Read the model definition and answer for the solid it produces. Units are mm, in the model's axes. Coordinates: 2 decimals unless noted, no trailing zeros. Write each loop counter-clockwise with the first axis right and the second up, starting at its lowest first coordinate (ties: lowest second). Pieces come first, ordered by that corner, then holes. Notation, with made-up numbers: (67, -4) -> (123, -4) arc R11 cw to (123, 11) -> close; hole circle Ø4 at (36, 5). An arc over 180 degrees is marked (long way). One line per item, written item: value. Start each with the question number.
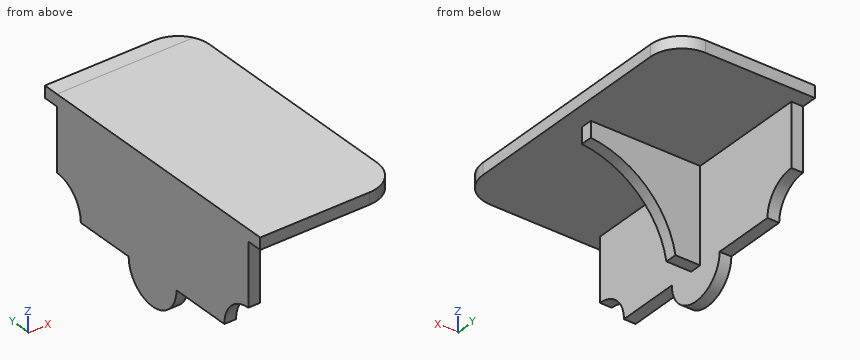
from build123d import *

# Parameters (mm, degrees)
F0_W      = 203.2
F0_H      = 9.525
F0_W_2    = 12.7
F1_DEPTH  = 114.3
F2_DEPTH  = 9.525
F3_W      = 9.525
F3_H      = 76.2
F4_DEPTH  = 88.9
F6_DEPTH  = 119.0635
F8_DEPTH  = 9.526
F10_DEPTH = 9.6059256377


with BuildPart() as f1:
    # F0 (on Right) → F1 (new body)
    with BuildSketch(Plane.YZ):
        with Locations((-2.4829334736, 39.2448874779)):
            Rectangle(F0_W, F0_H)
        Polygon((99.1170665264, 44.0073874779), (99.1170665264, 34.4823874779), (111.8170665264, 34.4823874779), (111.8170665264, 44.0873131156), align=None)
        with Locations((-110.4329334736, 39.2448874779)):
            Rectangle(F0_W_2, F0_H)
    extrude(amount=F1_DEPTH)

    # F0 (on Right) → F2 (join)
    with BuildSketch(Plane.YZ):
        Polygon((99.1170665264, 34.4823874779), (-104.0829334736, 34.4823874779), (-104.0829334736, -41.7176125221), (-27.8829334736, -41.7176125221), (22.9170665264, -41.7176125221), (99.1170665264, -41.7176125221), align=None)
        with BuildLine():
            Line((22.9170665264, -41.7176125221), (-27.8829334736, -41.7176125221))
            ThreePointArc((-27.8829334736, -41.7176125221), (-2.4829334736, -67.1176125221), (22.9170665264, -41.7176125221))
        make_face()
    extrude(amount=F2_DEPTH)

    # F3 (on face) → F4 (join)
    with BuildSketch(Plane.YZ.offset(9.525)):
        with Locations((-2.4829334736, -3.6176125221)):
            Rectangle(F3_W, F3_H)
    extrude(amount=F4_DEPTH)

    # F5 (on face) → F6 (cut, through all)
    with BuildSketch(Plane(origin=(0, 2.2795665264, 0), x_dir=(-1, 0, 0), z_dir=(0, 1, 0))):
        with BuildLine():
            ThreePointArc((-29.6407867546, -41.7176125221), (-53.2038437376, 1.6792308985), (-98.425, 21.5173431966))
            Line((-98.425, 21.5173431966), (-98.425, -41.7176125221))
            Line((-98.425, -41.7176125221), (-29.6407867546, -41.7176125221))
        make_face()
    extrude(amount=-F6_DEPTH, mode=Mode.SUBTRACT)

    # F7 (on face) → F8 (cut, through all)
    with BuildSketch(Plane.YZ.offset(9.525)):
        with BuildLine():
            Line((-104.0829334736, -41.7176125221), (-78.6829334736, -41.7176125221))
            ThreePointArc((-78.6829334736, -41.7176125221), (-86.1224212314, -23.75710028), (-104.0829334736, -16.3176125221))
            Line((-104.0829334736, -16.3176125221), (-104.0829334736, -41.7176125221))
        make_face()
        with BuildLine():
            Line((99.1170665264, -41.7176125221), (99.1170665264, -16.3176125221))
            ThreePointArc((99.1170665264, -16.3176125221), (81.1565542843, -23.75710028), (73.7170665264, -41.7176125221))
            Line((73.7170665264, -41.7176125221), (99.1170665264, -41.7176125221))
        make_face()
    extrude(amount=-F8_DEPTH, mode=Mode.SUBTRACT)

    # F9 (on face) → F10 (cut, through all)
    with BuildSketch(Plane(origin=(0, 0, 34.4823874779), x_dir=(1, 0, 0), z_dir=(0, 0, -1))):
        with BuildLine():
            ThreePointArc((88.9, 116.7829334736), (106.8605122421, 109.3434457157), (114.3, 91.3829334736))
            Line((114.3, 91.3829334736), (114.3, 116.7829334736))
            Line((114.3, 116.7829334736), (89.5812958479, 116.7829334736))
            Line((89.5812958479, 116.7829334736), (88.9, 116.7829334736))
        make_face()
        with BuildLine():
            Line((114.3, -111.8170665264), (114.3, -86.4170665264))
            ThreePointArc((114.3, -86.4170665264), (106.8605122421, -104.3775787686), (88.9, -111.8170665264))
            Line((88.9, -111.8170665264), (95.8859026432, -111.8170665264))
            Line((95.8859026432, -111.8170665264), (114.3, -111.8170665264))
        make_face()
    extrude(amount=-F10_DEPTH, mode=Mode.SUBTRACT)


solid = f1.part
1. A cutting plane is placed at B-B on x = 18.5. Give the vertices of the cut face in (y, z), then the cut area to 3 significant figures.
2. A cutting plane is placed at D-D on z = -8. Give the vertices of the cut face in (x, y) (1 decimal).
3. A cutting plane is placed at C-C on z = 8. Give the vertices of the cut face in (x, y) (3 decimals), then the cut area to 3 significant figures.
4. Given pin 1 (7.5 mm diameter, centred on x = 5.5, z = 18.5, fed in from -Y); pin 2 (1.5 mm diameter, centred on y = -48.5, z = -38, fed in from +X) (3 decimals); pin 3 (10.5 mm diameter, centred on x = 20, y = -2.5, fed in from -Z); pin 4 (23 mm diameter, centred on x = 57, z = -18.5, fed in from +Y), each flat-ended and moving along its own axis, determine where each tip first touches the part or whether it passes through.
5. Find the intervals of material crossed by probe 1 along Z at (x, y) = (67, 72.5); probe 2 along X at (y, z) = (31.5, 12) (3 decimals); probe 3 along Y at (x, z) = (74, 30.5), in increasing order. Write a range as from..to.
6. A cutting plane is placed at A-A on y = -43.5. Give the vertices of the cut face in (x, z) (3 decimals), then the cut area to 3 significant figures.
Derived:
1. outline: (-116.78, 34.48) -> (-7.25, 34.48) -> (-7.25, -41.72) -> (2.28, -41.72) -> (2.28, 34.48) -> (111.82, 34.48) -> (111.82, 44.09) -> (99.12, 44.01) -> (-116.78, 44.01) -> close
1. area: 2,900 mm2
2. outline: (0, -104.1) -> (9.5, -104.1) -> (9.5, -7.2) -> (44.3, -7.2) -> (44.3, 2.3) -> (9.5, 2.3) -> (9.5, 99.1) -> (0, 99.1) -> close
3. outline: (0, -104.083) -> (9.525, -104.083) -> (9.525, -7.245) -> (61.066, -7.245) -> (61.066, 2.28) -> (9.525, 2.28) -> (9.525, 99.117) -> (0, 99.117) -> close
3. area: 2,430 mm2
4. pin 1: stops at y = -104.08
4. pin 2: stops at x = 9.525
4. pin 3: stops at z = -41.72
4. pin 4: passes through
5. probe 1: z = 34.48..44.01
5. probe 2: x = 0..9.525
5. probe 3: y = -7.25..2.28
6. outline: (0, -41.718) -> (9.525, -41.718) -> (9.525, 34.482) -> (114.3, 34.482) -> (114.3, 44.007) -> (0, 44.007) -> close
6. area: 1,810 mm2
